Can you work these out from the drawing? Everything is in mm from the part's minimum corner. A direction names the side the tool comes from. Round coordinates to 2 decimals unless told otherwise and drop trailing zeros. Loops run counter-clockwise (first coordinate to the right, second up) from the corner with the lowest first, then second, coordinate; pieces in that order, holes last. Notation, with made-up numbers: (-21.5, -10.5) -> (3.5, -10.5) arc R21 cw to (3.5, -2.5) -> close; hole circle Ø8 at (18, 39.5). An arc over 180 degrees is marked (long way). One line per item, written item: value.
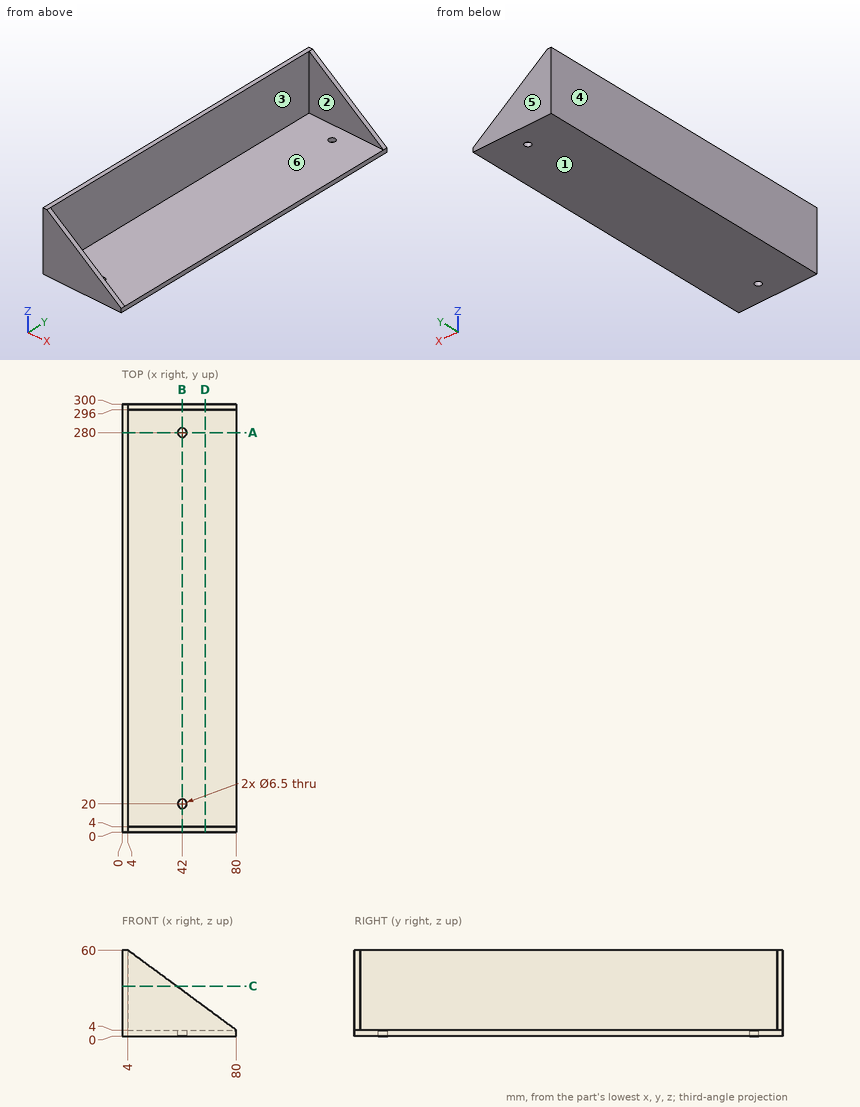
(1) Imagine slicing it at A-A on y = 280. Write out the boundary of the cut face in (x, z), then the cut area to 3 significant figures.
Results below:
outline: (0, 0) -> (38.75, 0) -> (38.75, 4) -> (4, 4) -> (4, 60) -> (0, 60) -> close; (45.25, 0) -> (80, 0) -> (80, 4) -> (45.25, 4) -> close
area: 518 mm²
(2) Imagine slicing it at C-C on z = 35. Write out the boundary of the cut face in (x, y).
Results below:
outline: (0, 0) -> (37.93, 0) -> (37.93, 4) -> (4, 4) -> (4, 296) -> (37.93, 296) -> (37.93, 300) -> (0, 300) -> close
(3) On a 3-axis mill with a long thin cutter (end or side, diameter ignored), from which of +Z, -Z, +X, -X, +Y, -Y can I reach the whole of each face in a straight line? I mean the marked faces 1 and 2. Say none if no direction works.
Results below:
face 1: -Z, +X, -X, +Y, -Y
face 2: +Z, +X
(4) Please list where these lines run through material, in increasing order: L1, parallel to Y at x = 42, z = 2; L2, parallel to X at y = 280, z = 2; L3, parallel to Y at x = 6, z = 12.5.
Results below:
L1: y = 0 to 16.75, 23.25 to 276.75, 283.25 to 300
L2: x = 0 to 38.75, 45.25 to 80
L3: y = 0 to 4, 296 to 300
(5) Imagine slicing it at B-B on x = 42. Write out the boundary of the cut face in (y, z), then the cut area to 3 significant figures.
Results below:
outline: (0, 0) -> (16.75, 0) -> (16.75, 4) -> (4, 4) -> (4, 32) -> (0, 32) -> close; (23.25, 0) -> (276.75, 0) -> (276.75, 4) -> (23.25, 4) -> close; (283.25, 0) -> (300, 0) -> (300, 32) -> (296, 32) -> (296, 4) -> (283.25, 4) -> close
area: 1,370 mm²
(6) For pin 1 Ø1.5 at (x, y) = (43, 107.5) entering from +Z; pin 2 Ø3 at (y, z) = (66, 47) entering from +X, each with a flat end and sliding along its axis, tell me the tip position at first contact or that it passes through.
Results below:
pin 1: stops at z = 4
pin 2: stops at x = 4
(7) Imagine slicing it at D-D on x = 58. Write out the boundary of the cut face in (y, z).
Results below:
outline: (0, 0) -> (300, 0) -> (300, 20.21) -> (296, 20.21) -> (296, 4) -> (4, 4) -> (4, 20.21) -> (0, 20.21) -> close
(8) We'd pull the mould along Y, two halves only. Please class the marked faces 3, 4, 5 and 6: +Y half, -Y half, draft (parallel to the pull), parting line (faces both ways), or undercut.
Results below:
face 3: undercut
face 4: draft
face 5: +Y half
face 6: undercut
